The figure shows three views and two pictorial views of one solid part (mm, origin at its lowest corner). Answer the questions. Coordinates: 2 decimals unless noted, no trailing zeros. Order: outer loops, then holes, each group sorted by start corner. A loop starts at its lowest first (then second) coordinate and runs counter-clockwise, first axis right, second up. Notation, with made-up numbers: (62, 56.5) -> (67, 56.5) arc R21 ccw to (67, 87.5) -> close; hole circle Ø4 at (-8, 79.25). An arc over 180 degrees is marked (long way). Return JSON: item names as keys, results as strings.
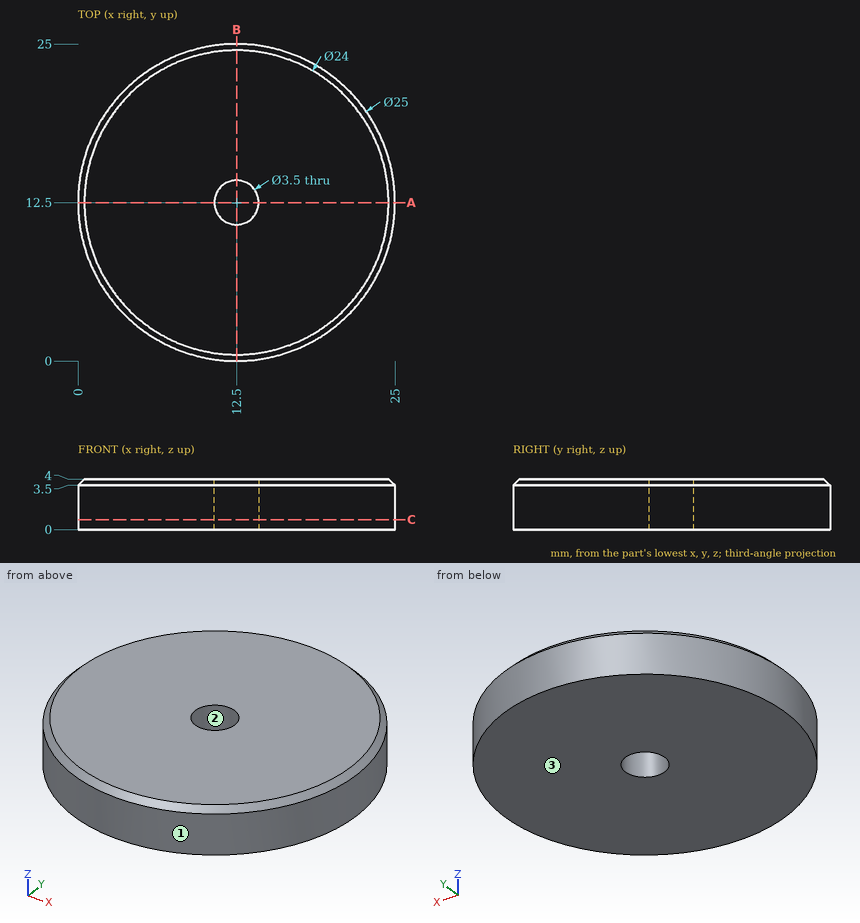
1. Each of these flat-tipped pins is pushed along its axis until it touches: pin 1 Ø8 at (x, y) = (18.5, 5.5) entering from -Z; pin 2 Ø1 at (y, z) = (10.5, 1) entering from +X. Where does it stop, or does it pass through?
Answer block:
{"pin 1": "stops at z = 0", "pin 2": "stops at x = 24.91"}
2. The part is cut by section C-C on z = 0.8. Give the vertices of the cut face in (x, y), and give its area (3 significant figures).
Answer block:
{"outline": "circle Ø25 at (12.5, 12.5); hole circle Ø3.5 at (12.5, 12.5)", "area": "481 mm2"}
3. Determine the mould class of the marked faces 1, 2 and 3 for opening direction X: pulls with the +X half, pulls with the -X half, needs draft (parallel to the pull), parting line crosses it, or undercut.
Answer block:
{"face 1": "parting line crosses it", "face 2": "undercut", "face 3": "needs draft"}
4. Consider line 1 (Y direction, x = 12.5, z = 1.55); line 2 (X direction, y = 12.75, z = 1.45); line 3 (Y direction, x = 9, z = 3.05). Determine where each line is inside the solid, lowest interval first. Write a range as from..to.
Answer block:
{"line 1": "y = 0..10.75, 14.25..25", "line 2": "x = 0..10.77, 14.23..25", "line 3": "y = 0.5..24.5"}
5. The part is cut by section A-A on y = 12.5. Give the vertices of the cut face in (x, z).
Answer block:
{"outline": "(0, 0) -> (10.75, 0) -> (10.75, 4) -> (0.5, 4) -> (0, 3.5) -> close; (14.25, 0) -> (25, 0) -> (25, 3.5) -> (24.5, 4) -> (14.25, 4) -> close"}
